Can you work these out from the model? Positions are in its coordinate system, mm. Round coordinates to 2 decimals unless told otherwise and drop trailing zeros. Order: outer loops, then holes, each group sorted by start corner. A loop starts at its lowest first (then second) coordinate and runs counter-clockwise, first axis right, second up.
from build123d import *

# Parameters (mm, degrees)
SKETCH1_W           = 88.9
SKETCH1_H           = 152.4
BOSS_EXTRUDE1_DEPTH = 38.1


with BuildPart() as part:
    # Sketch1 → Boss-Extrude1 (new body)
    with BuildSketch(Plane.XY):
        with Locations((44.45, 76.2)):
            Rectangle(SKETCH1_W, SKETCH1_H)
    extrude(amount=BOSS_EXTRUDE1_DEPTH)

    # SurfaceCut1
    split(bisect_by=Plane(origin=(37.404236669, 65.457414171, 87.276552228), x_dir=(0.9459459459459459, -0.19459459459459455, -0.2594594594594596), z_dir=(0.3243243243243244, 0.5675675675675675, 0.7567567567567568)), keep=Keep.BOTTOM)


solid = part.part
(1) I'm going to push a flat-ended pin straight in: pin 1 Ø3 at (x, y) = (9.5, 104.5) entering from -Z. Where does the tip first touch, or does it pass through?
(2) I want a section at A-A, the plane z = 25.5. List the corners of the cut face in (x, y) for me.
(3) Please list where these lines run through material, in increasing order: probe 1 along X at (y, z) = (122, 35.5); probe 2 along X at (y, z) = (124, 23); probe 3 along Y at (x, z) = (68, 18).
(4) I want a section at B-B, the plane x = 45.5. List the corners of the cut face in (y, z) for me.
Ans:
1. pin 1: stops at z = 0
2. outline: (0, 0) - (88.9, 0) - (88.9, 118.4) - (29.4, 152.4) - (0, 152.4) - close
3. probe 1: x = 0 to 59.27
3. probe 2: x = 0 to 84.93
3. probe 3: y = 0 to 140.34
4. outline: (0, 0) - (152.4, 0) - (152.4, 18.6) - (126.4, 38.1) - (0, 38.1) - close
